Source: three-view drawing plus pictorial views. Frame: mm from the lowest corner of the part. Coordinates: 2 decimals unless noted, no trailing zeros. Order: outer loops, then holes, each group sorted by start corner. A loop starts at its lowest first (then second) coordinate and runs counter-clockwise, first axis right, second up. Notation, with made-up numbers: (-16.5, 35.5) - (37.5, 35.5) arc R23 cw to (37.5, 56.5) - close; hole circle Ø11 at (53.25, 85.25). An arc over 180 degrees is marked (long way). One line per question, with ' | ' between items.
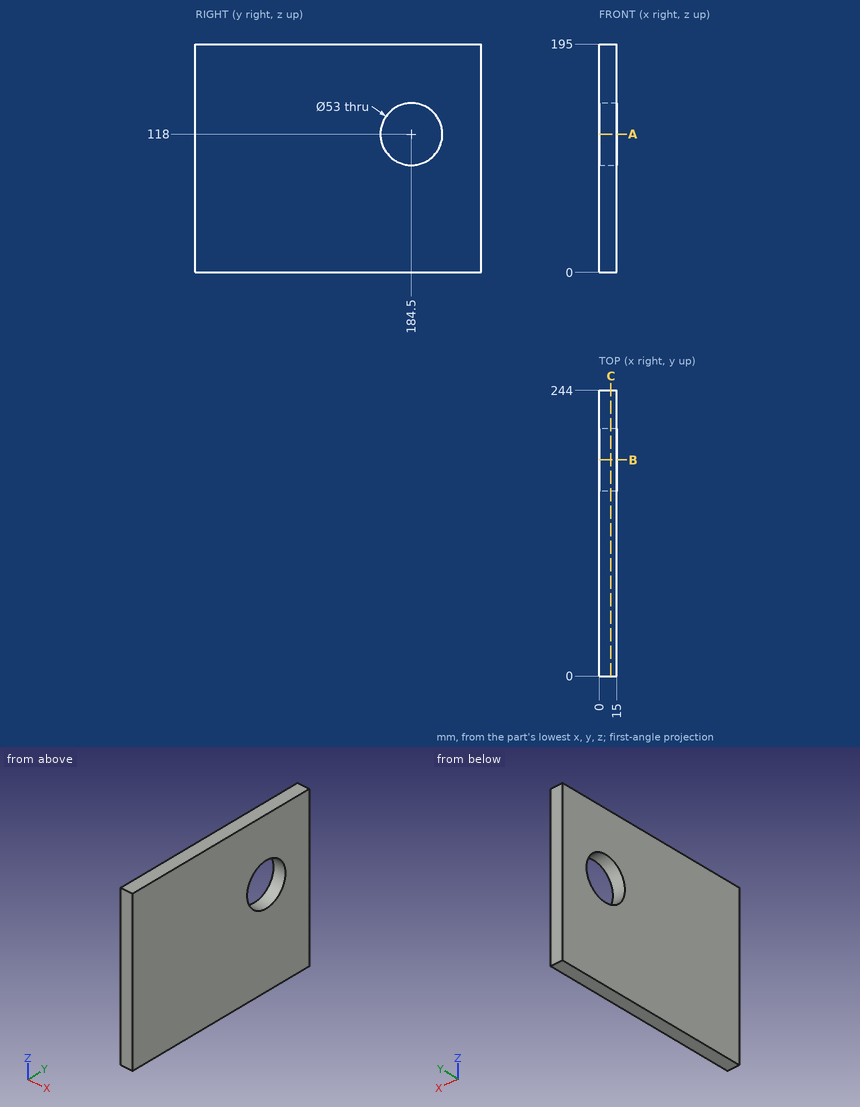
Item 1: Contact query for a flat-ended pin moving along its axis: P1, Ø1.5, axis at y = 189, z = 93.5, coming from the +X side. Output: stop coordinate, or through.
Data:
P1: through
Item 2: Section B-B on y = 184.5. Return the cut outline in (x, z).
Data:
outline: (0, 0) - (15, 0) - (15, 91.5) - (0, 91.5) - close; (0, 144.5) - (15, 144.5) - (15, 195) - (0, 195) - close
Item 3: Section C-C on x = 10. Return the cut outline in (y, z), and give its area (3 significant figures).
Data:
outline: (0, 0) - (244, 0) - (244, 195) - (0, 195) - close; hole circle Ø53 at (184.5, 118) | area: 45,400 mm^2
Item 4: Ray query, line 1 (Y direction, x = 7.5, z = 118); line 2 (Z direction, x = 13.5, y = 207.5); line 3 (Z direction, x = 1.75, y = 168). Return the intervals inside material, ascending.
Data:
line 1: 0 to 158, 211 to 244 | line 2: 0 to 104.84, 131.16 to 195 | line 3: 0 to 97.26, 138.74 to 195
Item 5: Section A-A on z = 118. Return the cut outline in (x, y), and give its area (4 significant figures).
Data:
outline: (0, 0) - (15, 0) - (15, 158) - (0, 158) - close; (0, 211) - (15, 211) - (15, 244) - (0, 244) - close | area: 2,865 mm^2
